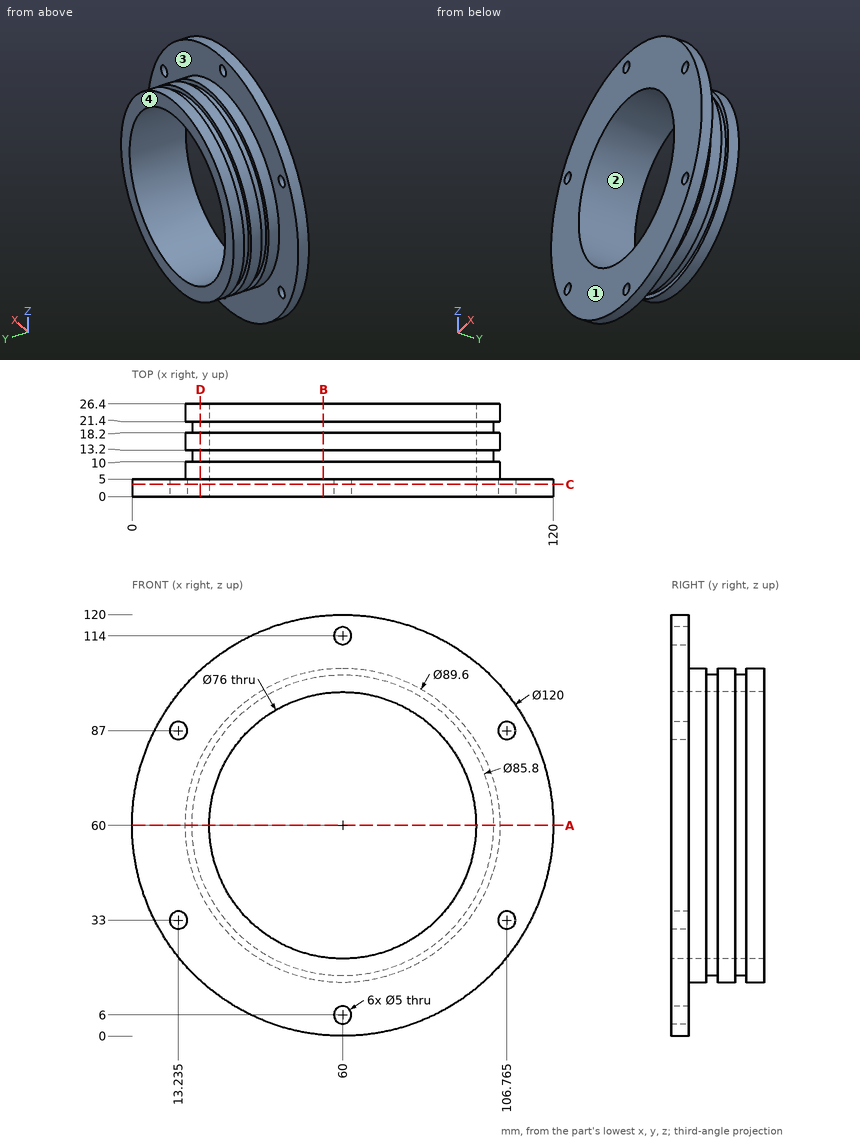
Verification items for this drawing (mm, ordinates from the low corner). A direction names the side the tool comes from. Coordinates: 2 decimals unless noted, no trailing zeros. Loops run counter-clockwise (first coordinate to the right, second up) from the corner with the lowest first, then second, coordinate; pieces in that order, holes last. Notation, with made-up numbers: (40, 73.5) -> (80, 73.5) arc R31 cw to (80, 109.5) -> close; hole circle Ø5 at (84, -3.75). An arc over 180 degrees is marked (long way). Answer in a Markdown table with one row per item. Add a question column.
1. Section check B-B, the plane x = 54.5. Enter the section's corners in (y, z).
2. Section check D-D, the plane x = 19.5. Enter the section's corners in (y, z), then the cut area to 3 significant figures.
3. Draft check along X on the marked faces 1 and 2. Enter one of: +X half, -X half, draft (parallel to the pull), parting line (faces both ways), or undercut.
4. Access from +Z, -Z, +X, -X, +Y, -Y to the whole of each face (thin tool, end or side, straight path). Record for the marked faces 3 and 4.
5. Material ranges on probe 1 along Y at (x, z) = (100.5, 76.5); probe 2 along X at (y, z) = (3.7, 87) (1 decimal); probe 3 along Y at (x, z) = (99, 88), recorded low to high. Write a range as [from, to].
6. Section check C-C, the plane y = 3.5. Enter the section's corners in (x, z) (1 decimal).
7. Section check A-A, the plane z = 60. Enter the section's corners in (x, y), then the cut area to 3 significant figures.
8. Depth check by flat-ended pin: P1, Ø8, axis at y = 16, z = 66.5, coming from the +X side; P2, Ø4, axis at x = 98, z = 102.5, coming from the +Y side; P3, Ø1, axis at x = 14.5, y = 4.5, coming from the -Z side (1 decimal); P4, Ø12, axis at x = 38.5, z = 101.5, coming from the +Y side. Enter the tip coordinate at first touch or a pass-through.
Derived:
| question | item | result |
|---|---|---|
| 1 | outline | (0, 0.25) -> (5, 0.25) -> (5, 15.54) -> (10, 15.54) -> (10, 17.45) -> (13.2, 17.45) -> (13.2, 15.54) -> (18.2, 15.54) -> (18.2, 17.45) -> (21.4, 17.45) -> (21.4, 15.54) -> (26.4, 15.54) -> (26.4, 22.4) -> (0, 22.4) -> close; (0, 97.6) -> (26.4, 97.6) -> (26.4, 104.46) -> (21.4, 104.46) -> (21.4, 102.55) -> (18.2, 102.55) -> (18.2, 104.46) -> (13.2, 104.46) -> (13.2, 102.55) -> (10, 102.55) -> (10, 104.46) -> (5, 104.46) -> (5, 119.75) -> (0, 119.75) -> close |
| 2 | outline | (0, 15.73) -> (5, 15.73) -> (5, 40.85) -> (10, 40.85) -> (10, 45.85) -> (13.2, 45.85) -> (13.2, 40.85) -> (18.2, 40.85) -> (18.2, 45.85) -> (21.4, 45.85) -> (21.4, 40.85) -> (26.4, 40.85) -> (26.4, 79.15) -> (21.4, 79.15) -> (21.4, 74.15) -> (18.2, 74.15) -> (18.2, 79.15) -> (13.2, 79.15) -> (13.2, 74.15) -> (10, 74.15) -> (10, 79.15) -> (5, 79.15) -> (5, 104.27) -> (0, 104.27) -> close |
| 2 | area | 1,200 mm² |
| 3 | face 1 | draft |
| 3 | face 2 | undercut |
| 4 | face 3 | +Y |
| 4 | face 4 | +Z, -Z, +X, -X, +Y |
| 5 | probe 1 | y = [0, 10], [13.2, 18.2], [21.4, 26.4] |
| 5 | probe 2 | x = [6.4, 10.7], [15.7, 33.3], [86.7, 104.3], [109.3, 113.6] |
| 5 | probe 3 | y = [0, 5] |
| 6 | outline | circle Ø120 at (60, 60); hole circle Ø5 at (13.2, 33); hole circle Ø5 at (13.2, 87); hole circle Ø76 at (60, 60); hole circle Ø5 at (60, 6); hole circle Ø5 at (60, 114); hole circle Ø5 at (106.8, 33); hole circle Ø5 at (106.8, 87) |
| 7 | outline | (0, 0) -> (22, 0) -> (22, 26.4) -> (15.2, 26.4) -> (15.2, 21.4) -> (17.1, 21.4) -> (17.1, 18.2) -> (15.2, 18.2) -> (15.2, 13.2) -> (17.1, 13.2) -> (17.1, 10) -> (15.2, 10) -> (15.2, 5) -> (0, 5) -> close; (98, 0) -> (120, 0) -> (120, 5) -> (104.8, 5) -> (104.8, 10) -> (102.9, 10) -> (102.9, 13.2) -> (104.8, 13.2) -> (104.8, 18.2) -> (102.9, 18.2) -> (102.9, 21.4) -> (104.8, 21.4) -> (104.8, 26.4) -> (98, 26.4) -> close |
| 7 | area | 487 mm² |
| 8 | P1 | stops at x = 104.73 |
| 8 | P2 | stops at y = 5 |
| 8 | P3 | stops at z = 20.3 |
| 8 | P4 | stops at y = 26.4 |
